Work out the finished part from the listing and answer in its coordinate system (mm). A direction names the side the tool comes from. Give positions to 0.01 mm unless a question says otherwise; leave off trailing zeros. Loops run counter-clockwise (first coordinate to the right, second up) from the corner with the lowest first, then second, coordinate; pieces in that order, holes last. Notation, with made-up numbers: (-11.75, -18) -> (43.25, -18) arc R17 ccw to (43.25, -14) -> close; hole circle Ø3 at (-33.5, 52). An arc over 180 degrees is marked (long way). Answer as CSV lines item,"result". Start each with the question number.
1. Find section A-A, the plane y = 0. Give the vertices of the cut face in (x, z) (3 decimals).
2. Flat-ended cylindrical pins translate along their axes: pin 1 Ø8 at (x, y) = (-10.16, 0) entering from -Z; pin 2 Ø4 at (x, y) = (8.5, 2) entering from +Z (3 decimals). Find the tip coordinate at first contact, or state that the pin passes through.
3. Find the intervals of material crossed by line 1 along Y through (x, z) = (10.5, 21.5); line 2 along Y through (x, z) = (10, 5); line 3 along Z through (x, y) = (0, 11), in increasing order.
4. Find section D-D, the plane z = 16. Give the vertices of the cut face in (x, y) (3 decimals), and give its area (3 significant figures).
5. Determine the mould class of faces 1 (the face through (19.05, 0, 16)), 2 (the face through (-15.03, 0.21, 20.79)), 3 (the face through (-19.05, 0, 16)) for opening direction X: +X half, -X half, draft (parallel to the pull), parting line (faces both ways), or undercut.
6. Find section B-B, the plane z = 25.4. Give the vertices of the cut face in (x, y) (3 decimals), and give its area (3 significant figures).
7. A tool of negligible diameter and unlimited length cuts with its end or side. For faces 4 (the face through (0, 19.05, 16)), 5 (the face through (14.8, 1.5, 20.8)), from which of +Z, -Z, +X, -X, +Y, -Y can it reach the whole face along a straight path? Write none if from no direction.
8. Find section C-C, the plane x = 10.16. Give the vertices of the cut face in (y, z) (3 decimals).
from build123d import *

# Parameters (mm, degrees)
F0_W           = 38.1
F0_H           = 38.1
F1_DEPTH       = 31.75
F3_D           = 3.4544
F5_D           = 5.5
F5_CBORE_D     = 9.75
F5_CBORE_DEPTH = 22.225


with BuildPart() as f1:
    # F0 (on Top) → F1 (new body)
    with BuildSketch(Plane.XY):
        Rectangle(F0_W, F0_H)
    extrude(amount=F1_DEPTH)

    # F3 (through all)
    with Locations(Plane.XZ.offset(19.05)):
        with Locations((0, 25.4)):
            Hole(F3_D / 2)

    # F5 (through all)
    with Locations(Plane.XY.offset(31.75)):
        with Locations((10.16, 0), (-10.16, 0)):
            CounterBoreHole(F5_D / 2, F5_CBORE_D / 2, F5_CBORE_DEPTH)


solid = f1.part
Resolved:
1,outline,"(-19.05, 0) -> (-12.91, 0) -> (-12.91, 9.525) -> (-15.035, 9.525) -> (-15.035, 31.75) -> (-19.05, 31.75) -> close; (-7.41, 0) -> (7.41, 0) -> (7.41, 9.525) -> (5.285, 9.525) -> (5.285, 31.75) -> (-5.285, 31.75) -> (-5.285, 9.525) -> (-7.41, 9.525) -> close; (12.91, 0) -> (19.05, 0) -> (19.05, 31.75) -> (15.035, 31.75) -> (15.035, 9.525) -> (12.91, 9.525) -> close; hole circle Ø3.454 at (0, 25.4)"
2,pin 1,"stops at z = 0"
2,pin 2,"stops at z = 9.525"
3,line 1,"y = -19.05 to -4.86, 4.86 to 19.05"
3,line 2,"y = -19.05 to -2.75, 2.75 to 19.05"
3,line 3,"z = 0 to 23.67, 27.13 to 31.75"
4,outline,"(-19.05, -19.05) -> (19.05, -19.05) -> (19.05, 19.05) -> (-19.05, 19.05) -> close; hole circle Ø9.75 at (-10.16, 0); hole circle Ø9.75 at (10.16, 0)"
4,area,"1,300 mm^2"
5,face 1,"+X half"
5,face 2,"undercut"
5,face 3,"-X half"
6,outline,"(-19.05, -19.05) -> (-1.727, -19.05) -> (-1.727, 19.05) -> (-19.05, 19.05) -> close; (1.727, -19.05) -> (19.05, -19.05) -> (19.05, 19.05) -> (1.727, 19.05) -> close; hole circle Ø9.75 at (-10.16, 0); hole circle Ø9.75 at (10.16, 0)"
6,area,"1,170 mm^2"
7,face 4,"+Z, -Z, +X, -X, +Y"
7,face 5,"+Z"
8,outline,"(-19.05, 0) -> (-2.75, 0) -> (-2.75, 9.525) -> (-4.875, 9.525) -> (-4.875, 31.75) -> (-19.05, 31.75) -> close; (2.75, 0) -> (19.05, 0) -> (19.05, 31.75) -> (4.875, 31.75) -> (4.875, 9.525) -> (2.75, 9.525) -> close"
